The figure shows three views and two pictorial views of one solid part (mm, origin at its lowest corner). Answer the questions. Coordinates: 2 decimals unless noted, no trailing zeros.
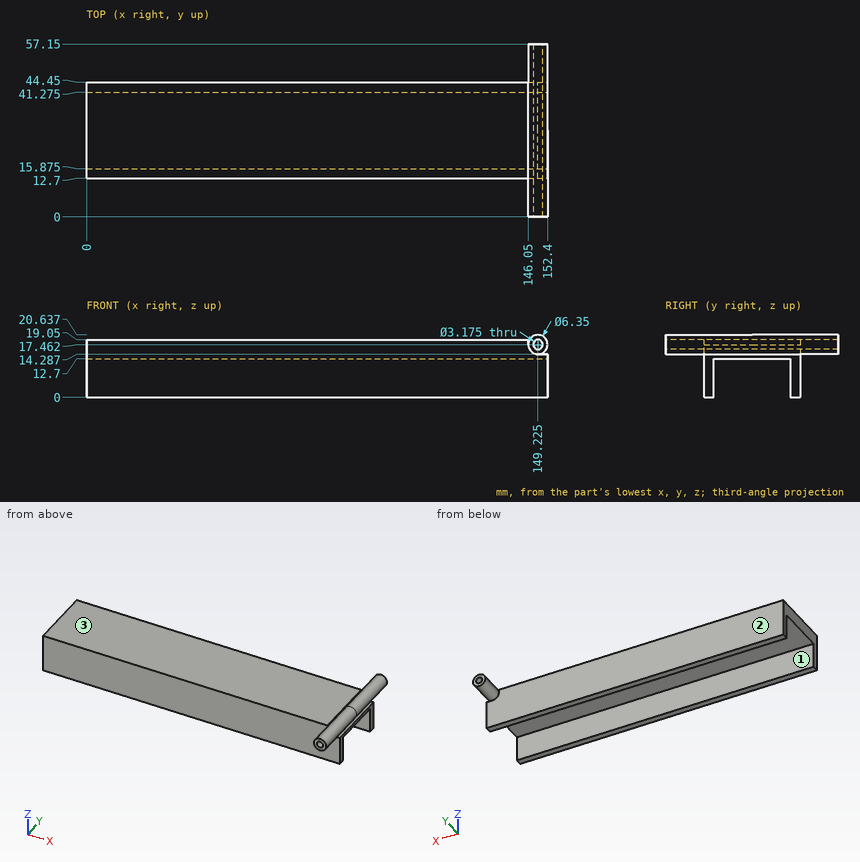
1. For a pull along Y with two mould halves and no side action, classify the marked faces 1, 2 and 3 as pulls with the +Y half, pulls with the -Y half, needs draft (parallel to the pull), parting line crosses it, or undercut.
Results found:
face 1: undercut
face 2: pulls with the +Y half
face 3: needs draft
2. Flat-ended cylindrical pins translate along their axes: P1, Ø1.6, axis at x = 151, y = 26, coming from the +Z side (1 decimal); P2, Ø10, axis at x = 51.5, z = 4, coming from the -Y side; P3, Ø0.8, axis at y = 32.5, z = 18, coming from the +X side. Find the tip coordinate at first contact, or state that the pin passes through.
Results found:
P1: stops at z = 20.5
P2: stops at y = 12.7
P3: stops at x = 152.4
3. Find the intervals of material crossed by L1, parallel to Y at x = 72.5, z = 13; L2, parallel to Z at x = 69.5, y = 16; L3, parallel to X at y = 34, z = 14.75 (1 decimal), in increasing order.
Results found:
L1: y = 12.7 to 44.45
L2: z = 12.7 to 19.05
L3: x = 0 to 150.9
